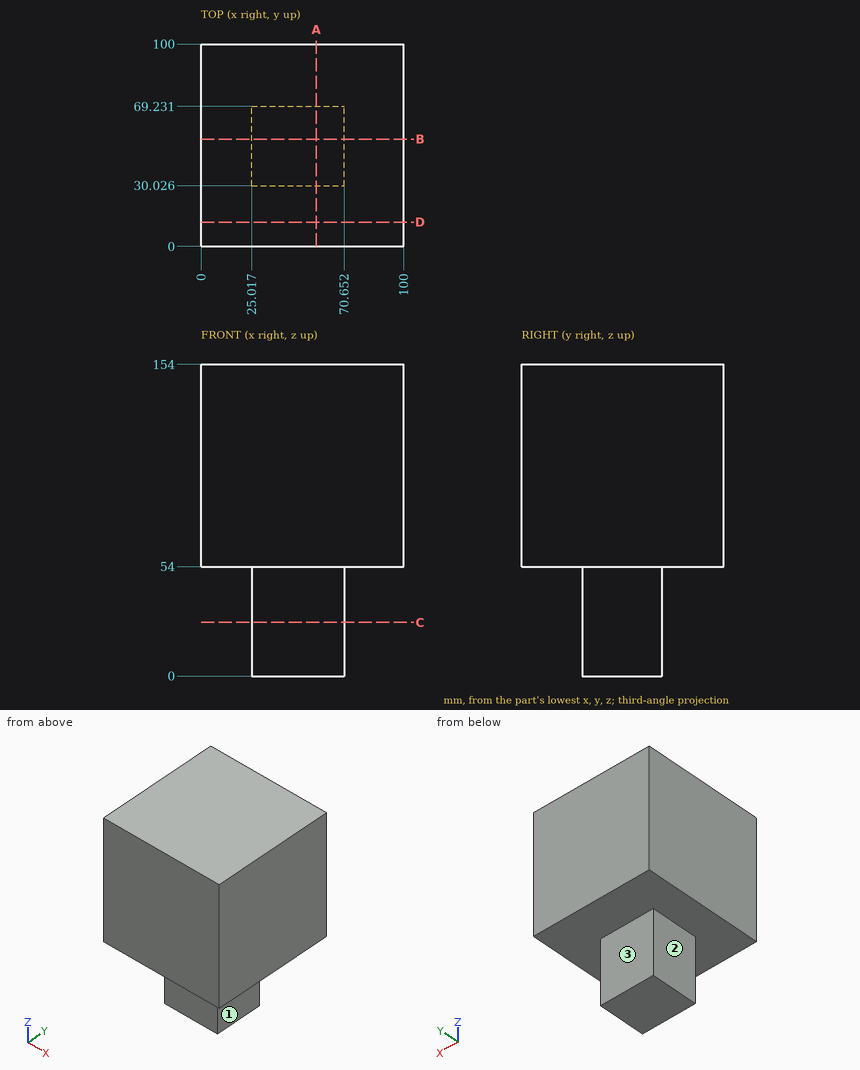
Print and shaded views of the part. All mm, measured from the part's lowest x, y and z. A direction names the side the tool comes from. Coordinates: 2 decimals unless noted, no trailing zeros. Order: outer loops, then holes, each group sorted by start corner. A loop starts at its lowest first (then second) coordinate and runs counter-clockwise, first axis right, second up.
(1) Slice it at C-C, the plane z = 26.5. Write the cut outline in (x, y).
Check sheet entries:
outline: (25.02, 30.03) - (70.65, 30.03) - (70.65, 69.23) - (25.02, 69.23) - close
(2) Pin check, flat tips, straight feed: pin 1 Ø4 at (x, z) = (86.5, 106) entering from -Y; pin 2 Ø1 at (x, y) = (17, 61.5) entering from -Z; pin 3 Ø13.5 at (x, z) = (57.5, 35) entering from +Y; pin 4 Ø19.5 at (y, z) = (41.5, 39.5) entering from +X. Stop position of each tip, or through.
Check sheet entries:
pin 1: stops at y = 0
pin 2: stops at z = 54
pin 3: stops at y = 69.23
pin 4: stops at x = 70.65
(3) Tool access for the marked faces 1, 2 and 3: list every direction of +Z, -Z, +X, -X, +Y, -Y with a clear straight run to the whole face (end or side of a thin tool).
Check sheet entries:
face 1: -Z, +X, +Y, -Y
face 2: -Z, -X, +Y, -Y
face 3: -Z, +X, -X, +Y
(4) Slice it at A-A, the plane x = 57. Write the cut outline in (y, z).
Check sheet entries:
outline: (0, 54) - (30.03, 54) - (30.03, 0) - (69.23, 0) - (69.23, 54) - (100, 54) - (100, 154) - (0, 154) - close
(5) Slice it at B-B, the plane y = 53. Write the cut outline in (x, z), and give its area (3 significant figures).
Check sheet entries:
outline: (0, 54) - (25.02, 54) - (25.02, 0) - (70.65, 0) - (70.65, 54) - (100, 54) - (100, 154) - (0, 154) - close
area: 12,500 mm2
(6) Slice it at D-D, the plane y = 12. Write the cut outline in (x, z), and give its area (3 significant figures).
Check sheet entries:
outline: (0, 54) - (100, 54) - (100, 154) - (0, 154) - close
area: 10,000 mm2
(7) Probe L1, parallel to Z at x = 19.5, y = 15.5; L2, parallel to X at y = 56.5, z = 17.5; L3, parallel to Y at x = 58, z = 7. List the from-to ranges inside material, lowest first.
Check sheet entries:
L1: z = 54 to 154
L2: x = 25.02 to 70.65
L3: y = 30.03 to 69.23
